Design review of the part built by this model. Coordinates are the model's own, in mm. Round coordinates to 2 decimals unless told otherwise and drop trailing zeros. Loops run counter-clockwise (first coordinate to the right, second up) from the corner with the lowest first, then second, coordinate; pieces in that order, holes last. Notation, with made-up numbers: M 65.25,-26 L 106.25,-26 A26 cw 106.25,1 Z; hole C -15,-16.75 d6. An arc over 180 degrees is marked long. Use a Markdown table: item, result.
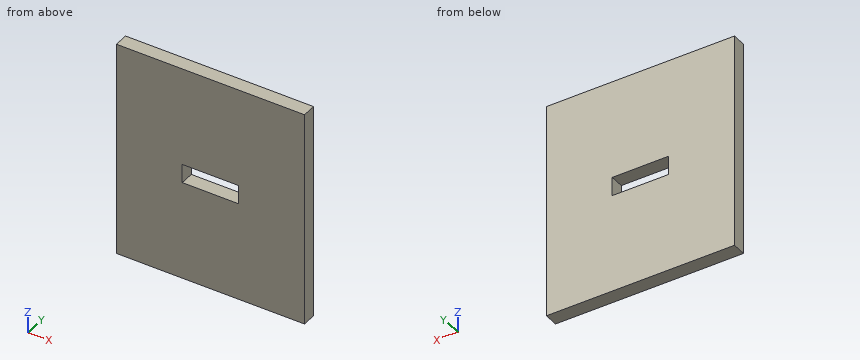
Autodesk Inventor part; units mm, degrees
ref_plane "YZ Plane" through (0, 0, 0) normal (1, 0, 0) x (0, 1, 0)
ref_plane "XZ Plane" through (0, 0, 0) normal (0, 1, 0) x (-1, 0, 0)
ref_plane "XY Plane" through (0, 0, 0) normal (0, 0, 1) x (1, 0, 0)
sketch "Sketch1" plane through (0, 0, 0) normal (0, 1, 0) x (-1, 0, 0)
  line L0 (0, 0) -> (0, -23)
  line L1 (0, -23) -> (20, -23)
  line L2 (20, -23) -> (20, 0)
  line L3 (16.0214, -11.5) -> (3.8301, -11.5) construction
  line L4 (20, 0) -> (0, 0)
  line L5 (13, -10.5) -> (7, -10.5)
  line L6 (7, -10.5) -> (7, -12.5)
  line L7 (7, -12.5) -> (13, -12.5)
  line L8 (13, -12.5) -> (13, -10.5)
  line L9 (10, -8) -> (10, -15) construction
  dimension "d0" = 23
  dimension "d10" = 20
  dimension "d13" = 10
  dimension "d14" = 2
  dimension "d15" = 6
extrude "Extrusion4" add sketch "Sketch1" along normal blind 1.5
properties part number "Distance_test_adaptor_slit_2mm"
1. Take a section at A-A on y = 0.8. Give the boundary of the cut face in (x, z), and give its area (3 significant figures).
Check values:
| item | result |
|---|---|
| outline | M -20,-23 L 0,-23 L 0,0 L -20,0 Z; hole M -13,-12.5 L -7,-12.5 L -7,-10.5 L -13,-10.5 Z |
| area | 448 mm² |
2. Wall thickness on line 1 along Z through (x, y) = (-11, 1.35): over which ranges is the line inside the solid? List them lowest first. Write a range as from..to.
Check values:
| item | result |
|---|---|
| line 1 | z = -23..-12.5, -10.5..0 |
3. Take a section at B-B on z = -12.25. Give the boundary of the cut face in (x, y), and give its area (3 significant figures).
Check values:
| item | result |
|---|---|
| outline | M -20,0 L -13,0 L -13,1.5 L -20,1.5 Z; M -7,0 L 0,0 L 0,1.5 L -7,1.5 Z |
| area | 21.0 mm² |
